Geometry check sheet. Reference: the model listing, model coordinates, mm. A direction names the side the tool comes from. Give positions to 0.01 mm unless a question says otherwise; leave off trailing zeros. Loops run counter-clockwise (first coordinate to the right, second up) from the corner with the lowest first, then second, coordinate; pieces in that order, holes last. Notation, with made-up numbers: (85, 76) -> (90, 76) arc R15 cw to (90, 102) -> close; hole circle Ø10 at (12, 74). An arc over 180 degrees is marked (long way). Write item = value, one per line.
```python
from build123d import *

# Parameters (mm, degrees)
CROQUIS1_R              = 20.75
SALIENTE_EXTRUIR1_DEPTH = 10


with BuildPart() as part:
    # Croquis1 → Saliente-Extruir1 (new body)
    with BuildSketch(Plane.XY):
        with BuildLine():
            ThreePointArc((-4.78021978, 21.218199708), (-0.225829084, -21.748827583), (5.21978022, 21.114364647))
            Line((5.21978022, 21.114364647), (5.21978022, 22.218199708))
            Line((5.21978022, 22.218199708), (-4.78021978, 22.218199708))
            Line((-4.78021978, 22.218199708), (-4.78021978, 21.218199708))
        make_face()
        Circle(CROQUIS1_R, mode=Mode.SUBTRACT)
        with BuildLine():
            ThreePointArc((-17.300656672, 13.181417933), (-13.806881781, 16.805728651), (-9.57346835, 19.529751759))
            Line((-9.57346835, 19.529751759), (-10.28299985, 20.375338473))
            Line((-10.28299985, 20.375338473), (-17.943444281, 13.947462376))
            Line((-17.943444281, 13.947462376), (-17.300656672, 13.181417933))
        make_face()
        with BuildLine():
            Line((18.280167114, 13.664918372), (10.619722682, 20.092794469))
            Line((10.619722682, 20.092794469), (9.976935073, 19.326750026))
            ThreePointArc((9.976935073, 19.326750026), (14.15287201, 16.515408377), (17.570635613, 12.819331657))
            Line((17.570635613, 12.819331657), (18.280167114, 13.664918372))
        make_face()
        with BuildLine():
            ThreePointArc((-21.725924031, -1.023095788), (-21.379199214, 3.999042508), (-19.887184682, 8.806950973))
            Line((-19.887184682, 8.806950973), (-20.974250008, 8.99862992))
            Line((-20.974250008, 8.99862992), (-22.710731784, -0.84944761))
            Line((-22.710731784, -0.84944761), (-21.725924031, -1.023095788))
        make_face()
        with BuildLine():
            Line((21.050578877, 8.565747391), (20.065771124, 8.392099213))
            ThreePointArc((20.065771124, 8.392099213), (21.457628831, 3.554246044), (21.699995328, -1.474009086))
            Line((21.699995328, -1.474009086), (22.787060653, -1.282330139))
            Line((22.787060653, -1.282330139), (21.050578877, 8.565747391))
        make_face()
        with BuildLine():
            Line((21.631635264, -6.969308089), (20.76560986, -6.469308089))
            ThreePointArc((20.76560986, -6.469308089), (18.722122647, -11.069987515), (15.675686059, -15.077644596))
            Line((15.675686059, -15.077644596), (16.631635264, -15.629562127))
            Line((16.631635264, -15.629562127), (21.631635264, -6.969308089))
        make_face()
        with BuildLine():
            ThreePointArc((-15.98539008, -14.748891619), (-18.947951731, -10.678840068), (-20.895466279, -6.036720051))
            Line((-20.895466279, -6.036720051), (-21.851415483, -6.588637582))
            Line((-21.851415483, -6.588637582), (-16.851415483, -15.248891619))
            Line((-16.851415483, -15.248891619), (-15.98539008, -14.748891619))
        make_face()
        with BuildLine():
            Line((-3.107134595, -22.513209767), (-2.765114452, -21.573517146))
            ThreePointArc((-2.765114452, -21.573517146), (-7.65074705, -20.359974695), (-12.126526978, -18.055742673))
            Line((-12.126526978, -18.055742673), (-12.504060803, -19.093008334))
            Line((-12.504060803, -19.093008334), (-3.107134595, -22.513209767))
        make_face()
        with BuildLine():
            Line((12.091009102, -19.243346858), (11.748988958, -18.303654238))
            ThreePointArc((11.748988958, -18.303654238), (7.226327204, -20.514450886), (2.316549068, -21.626282631))
            Line((2.316549068, -21.626282631), (2.694082894, -22.663548292))
            Line((2.694082894, -22.663548292), (12.091009102, -19.243346858))
        make_face()
    extrude(amount=SALIENTE_EXTRUIR1_DEPTH)


solid = part.part
```
Item 1: Gauge pin test, flat ends, axial feed: pin 1 (0.5 mm diameter, centred on y = 22, z = 2.5, fed in from -X); pin 2 (0.6 mm diameter, centred on y = 22, z = 2.5, fed in from +X); pin 3 (4 mm diameter, centred on y = 8.5, z = 3, fed in from -X). Record the tip position at first contact, or that the pin passes through.
Answer:
pin_1 = -4.78
pin_2 = 5.22
pin_3 = -21.41
Item 2: Section check A-A, the plane x = 0. Record the cut outline in (y, z), plus the area to 3 significant figures.
Answer:
outline = (-21.75, 0) -> (-20.75, 0) -> (-20.75, 10) -> (-21.75, 10) -> close; (20.75, 0) -> (22.22, 0) -> (22.22, 10) -> (20.75, 10) -> close
area = 24.7 mm^2
Item 3: Draft check along Y on faces 1 (the cylindrical face through (18.965, 10.648, 4.93)), 2 (the flat face through (-19.386, -10.858, 4.93)), 3 (the flat face through (-20.42, 8.9, 4.93)). Enter one of: +Y half, -Y half, draft (parallel to the pull), parting line (faces both ways), or undercut.
Answer:
face_1 = undercut
face_2 = -Y half
face_3 = +Y half
Item 4: Tool access check on faces 4 (the flat face through (7.327, -20.977, 4.93)), 5 (the flat face through (-12.313, -18.567, 4.93)), 6 (the flat face through (-4.78, 22, 5)), 7 (the flat face through (5.22, 22, 5)), 8 (the flat face through (20.57, 8.48, 4.93)). Record the directions out of +Z, -Z, +X, -X, +Y, -Y that give a thin tool (end or side, any length) a straight path to the whole face; none if there is none.
Answer:
face_4 = +Z, -Z, +X, -Y
face_5 = +Z, -Z, -X
face_6 = +Z, -Z, -X, +Y
face_7 = +Z, -Z, +X, +Y
face_8 = +Z, -Z, +Y
Item 5: Thickness scan on L1, parallel to Y at x = 0, z = 4.5; L2, parallel to X at y = 3, z = 1; L3, parallel to X at y = 15.5, z = 5.75. Record the ranges inside material, lowest first. Write a range as [from, to].
Answer:
L1 = [-21.75, -20.75], [20.75, 22.22]
L2 = [-22.03, -20.53], [20.53, 22.03]
L3 = [-16.09, -13.8], [13.8, 16.09]
Item 6: Section check B-B, the plane y = 0. Record the cut outline in (x, z), plus the area to 3 significant figures.
Answer:
outline = (-22.56, 0) -> (-20.75, 0) -> (-20.75, 10) -> (-22.56, 10) -> close; (20.75, 0) -> (22.56, 0) -> (22.56, 10) -> (20.75, 10) -> close
area = 36.2 mm^2
